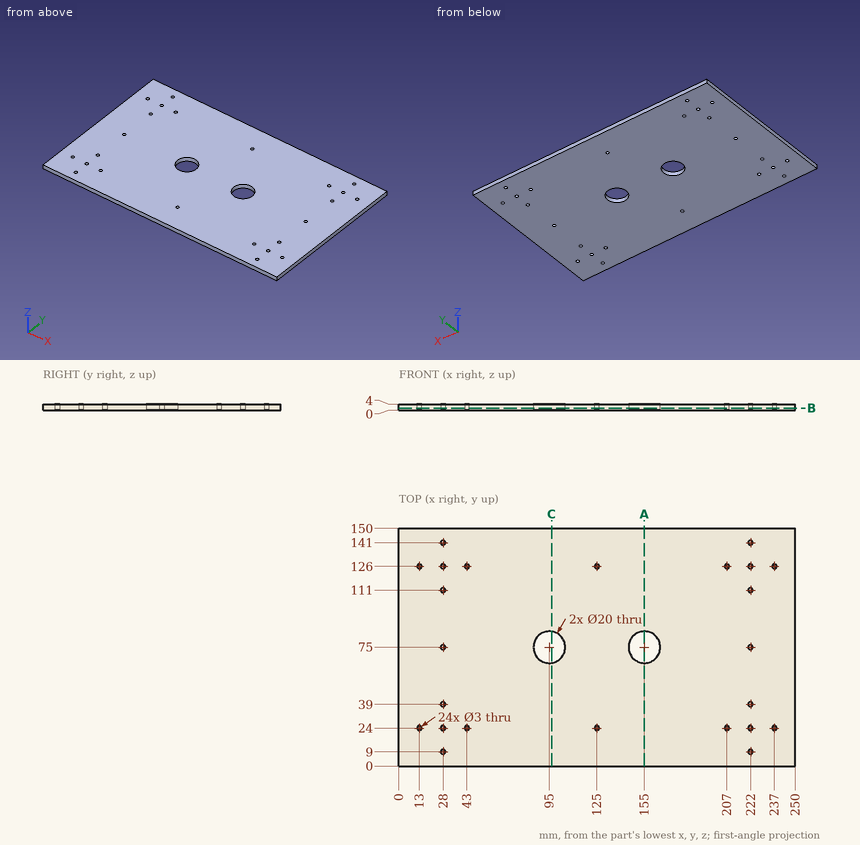
Answer from the drawing. Dimensions are ordinates in mm from the lowest x, y and z of the part. Give positions to 0.01 mm unless a question says otherwise; leave off trailing zeros. Loops run counter-clockwise (first coordinate to the right, second up) from the corner with the lowest first, then second, coordinate; pieces in that order, holes last. Notation, with made-up numbers: M -36,23.25 L 11,23.25 A15 cw 11,34.25 Z; hole C 13,17 d6. An arc over 180 degrees is marked long. One line per item, written item: value.
Q1. A cutting plane is placed at A-A on x = 155. Determine the outline of the cut face in (y, z).
Working result:
outline: M 0,0 L 65,0 L 65,4 L 0,4 Z; M 85,0 L 150,0 L 150,4 L 85,4 Z
Q2. A flat-ended cylindrical pin translates along its axis: P1, Ø2.5, axis at x = 222, y = 111, coming from the -Z side. Find the tip coordinate at first contact, or state that the pin passes through.
Working result:
P1: passes through
Q3. Find the intervals of material crossed by line 1 (Y direction, x = 13, z = 2.2); line 2 (X direction, y = 9, z = 1.8); line 3 (X direction, y = 70, z = 1.85), in increasing order. Write a range as from..to.
Working result:
line 1: y = 0..22.5, 25.5..124.5, 127.5..150
line 2: x = 0..26.5, 29.5..220.5, 223.5..250
line 3: x = 0..86.34, 103.66..146.34, 163.66..250
Q4. A cutting plane is placed at C-C on x = 96.5. Determine the outline of the cut face in (y, z), then the cut area to 3 significant figures.
Working result:
outline: M 0,0 L 65.11,0 L 65.11,4 L 0,4 Z; M 84.89,0 L 150,0 L 150,4 L 84.89,4 Z
area: 521 mm^2
Q5. A cutting plane is placed at B-B on z = 1.4. Give the number of separate pieces and of enclosed holes in the cut face, then the cut area to 3 significant figures.
Working result:
separate pieces: 1
enclosed holes: 26
area: 36,700 mm^2
